```python
from build123d import *

# Parameters (mm, degrees)
DODANIE_WYCI_GNI_CIE1_DEPTH = 10
SZKIC2_R                    = 2
WYTNIJ_WYCI_GNI_CIE1_DEPTH  = 10


with BuildPart() as part:
    # Szkic1 → Dodanie-wyciągnięcie1 (new body)
    with BuildSketch(Plane(origin=(0, 0, 502.999346089), x_dir=(-1, 0, 0), z_dir=(0, 0, -1))):
        with BuildLine():
            Line((-929.814034739, -322.668005597), (-970.58269303, -291.759349877))
            Line((-970.58269303, -291.759349877), (-980.58269303, -291.759349877))
            Line((-980.58269303, -291.759349877), (-980.58269303, -293.759349877))
            Line((-980.58269303, -293.759349877), (-971.255135855, -293.759349877))
            Line((-971.255135855, -293.759349877), (-930.899175905, -324.355119388))
            add(Edge.make_bspline(
                [(-929.814034739, -322.668005597), (-930.214433706, -323.196133667), (-930.577577349, -323.759219062), (-930.899175905, -324.355119388)],
                knots=[0.163263648, 0.163263648, 0.163263648, 0.163263648, 0.18460997, 0.18460997, 0.18460997, 0.18460997], degree=3, weights=[0.560185558, 0.55031088, 0.54165131, 0.534206848]))
        make_face()
    extrude(amount=DODANIE_WYCI_GNI_CIE1_DEPTH)

    # Szkic2 → Wytnij-wyciągnięcie1 (cut)
    with BuildSketch(Plane(origin=(0, -293.759349877, 0), x_dir=(-1, 0, 0), z_dir=(0, -1, 0))):
        with Locations((-975.58269303, -497.999346089)):
            Circle(SZKIC2_R)
    extrude(amount=-WYTNIJ_WYCI_GNI_CIE1_DEPTH, mode=Mode.SUBTRACT)


solid = part.part
```
Geometry: final body of the model. Coordinates: model frame, mm. A direction names the side the tool comes from. Give positions to 0.01 mm unless a question says otherwise; leave off trailing zeros. Loops run counter-clockwise (first coordinate to the right, second up) from the corner with the lowest first, then second, coordinate; pieces in that order, holes last. Notation, with made-up numbers: (40.25, 39.25) -> (74.25, 39.25) arc R11 ccw to (74.25, 50.25) -> close; hole circle Ø2 at (-28, 52). An arc over 180 degrees is marked (long way). Use CSV: the item, a comma, the result in double quotes.
(1) Pull-direction query (X, two-part tool) for faces 1 (the face through (977.58, -292.77, 497.91)), 2 (the face through (973, -291.759, 498)), 3 (the face through (949.91, -307.43, 498.07)); classes: released by +X, released by -X, zero draft, split by the parting line, or undercut.
From the geometry:
face 1,"undercut"
face 2,"zero draft"
face 3,"released by -X"
(2) Access query for faces 4 (the face through (980.583, -293, 498)), 5 (the face through (978, -293.759, 498)). Directions: +Z, -Z, +X, -X, +Y, -Y. A direction counts if a zero-diameter tool reaches every point of the face in a straight line with its end or side. Return the directions, or none.
From the geometry:
face 4,"+Z, -Z, +X, +Y, -Y"
face 5,"+Z, -Z, +X, -Y"
(3) Ray query, line 1 along Y through (x, z) = (968.5, 501.75); line 2 along X through (y, z) = (-306, 495.25); line 3 along Y through (x, z) = (948.5, 501.25). Return the intervals inside material, ascending. Write a range as [from, to].
From the geometry:
line 1,"[-295.85, -293.34]"
line 2,"[951.8, 955.11]"
line 3,"[-311.01, -308.5]"
(4) Cut plane A-A (y = -312). Output: boundary loops of the cut face in (x, z).
From the geometry:
outline,"(943.89, 493) -> (947.2, 493) -> (947.2, 503) -> (943.89, 503) -> close"
(5) First-contact query: P1, Ø1.5, axis at y = -309, z = 501, coming from the -X side; P2, Ø4, axis at y = -319, z = 495, coming from the -X side; P3, Ø2, axis at y = -305.5, z = 499, coming from the +X side. Flat tips, straight axial feed; report the tip coordinate or a pass-through.
From the geometry:
P1,"x = 946.85"
P2,"x = 932.01"
P3,"x = 957.09"
(6) Cut plane B-B (x = 953.5). Output: boundary loops of the cut face in (y, z).
From the geometry:
outline,"(-307.22, 493) -> (-304.71, 493) -> (-304.71, 503) -> (-307.22, 503) -> close"
